Part model, mm, in its own coordinate system. Round coordinates to 2 decimals unless told otherwise and drop trailing zeros. Write each loop counter-clockwise with the first axis right and the second up, starting at its lowest first coordinate (ties: lowest second). Pieces come first, ordered by that corner, then holes. Notation, with made-up numbers: (-20, -16.5) -> (21, -16.5) arc R34 cw to (21, 15.5) -> close; hole circle Ø10 at (39, 57.5). An arc over 180 degrees is marked (long way). Return JSON: item names as keys, results as strings. Group by question number.
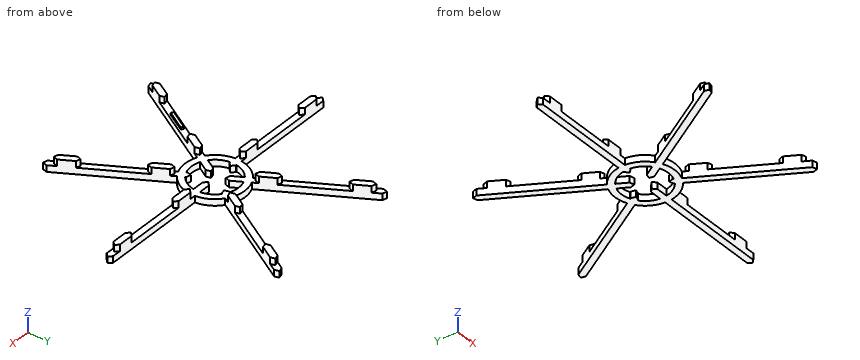
```python
from build123d import *

# Parameters (mm, degrees)
F1_DEPTH = 3
F4_DEPTH = 3
F5_COUNT = 3
F5_ANGLE = 240
F7_DEPTH = 1
F8_R     = 14
F8_R_2   = 11
F9_DEPTH = 3


# Not quite as in the source:
# - a feature names something its author has since deleted; it is built from what else it names


with BuildPart() as f1:
    # F0 (on Top) → F1 (new body)
    with BuildSketch(Plane.XY):
        Polygon((-2, -3.4641016151), (-4.0490381057, -4.0131397208), (-32.5490381057, -53.3765877365), (-32, -55.4256258422), (-29.9509618943, -54.8765877365), (-1.4509618943, -5.5131397208), align=None)
    extrude(amount=F1_DEPTH)

    # F3 (on face) → F4, piece 2 (join)
    with BuildSketch(Plane.XY.offset(3)):
        Polygon((-27.0490381057, -43.8503082949), (-30.5490381057, -49.9124861214), (-30, -51.9615242271), (-27.9509618943, -51.4124861214), (-24.4509618943, -45.3503082949), (-25, -43.3012701892), align=None)
        Polygon((-9.5490381057, -13.5394191624), (-13.0490381057, -19.6015969889), (-12.5, -21.6506350946), (-10.4509618943, -21.1015969889), (-6.9509618943, -15.0394191624), (-7.5, -12.9903810568), align=None)
    extrude(amount=F4_DEPTH)


with BuildPart() as f1b:
    # F0 (on Top) → F1, piece 2 (new body)
    with BuildSketch(Plane.XY):
        Polygon((-10.5, 1.5), (-62.5, 1.5), (-64, 0), (-62.5, -1.5), (-10.5, -1.5), (-9, 0), align=None)
    extrude(amount=F1_DEPTH)

    # F3 (on face) → F4 (join)
    with BuildSketch(Plane.XY.offset(3)):
        Polygon((-51.5, 1.5), (-58.5, 1.5), (-60, 0), (-58.5, -1.5), (-51.5, -1.5), (-50, 0), align=None)
        Polygon((-16.5, 1.5), (-23.5, 1.5), (-25, 0), (-23.5, -1.5), (-16.5, -1.5), (-15, 0), align=None)
    extrude(amount=F4_DEPTH)


with BuildPart() as f5_1:
    # F5: instance of F1
    add(f1.part.rotate(Axis((0, 0, 0.1916177571), (0, 0, -1)), 1 * F5_ANGLE / (F5_COUNT - 1)))


with BuildPart() as f5_2:
    # F5: instance of F1
    add(f1.part.rotate(Axis((0, 0, 0.1916177571), (0, 0, -1)), 2 * F5_ANGLE / (F5_COUNT - 1)))


with BuildPart() as f5_3:
    # F5: instance of F1b
    add(f1b.part.rotate(Axis((0, 0, 0.1916177571), (0, 0, -1)), 1 * F5_ANGLE / (F5_COUNT - 1)))


with BuildPart() as f5_4:
    # F5: instance of F1b
    add(f1b.part.rotate(Axis((0, 0, 0.1916177571), (0, 0, -1)), 2 * F5_ANGLE / (F5_COUNT - 1)))


with BuildPart() as f1_1:
    add(f1.part)

    # F6 (on face) → F7 (join)
    with BuildSketch(Plane.XY.offset(3)):
        Polygon((-15.7303847577, -28.445825623), (-16.7696152423, -27.845825623), (-21.7696152423, -36.5060796608), (-20.7303847577, -37.1060796608), align=None)
    extrude(amount=F7_DEPTH)

    add(f1b.part)  # F9 merges F1b

    add(f5_1.part)  # F9 merges F5_1

    add(f5_2.part)  # F9 merges F5_2

    add(f5_3.part)  # F9 merges F5_3

    add(f5_4.part)  # F9 merges F5_4
    # F8 (on Top) → F9 (join)
    with BuildSketch(Plane.XY):
        Circle(F8_R)
        Circle(F8_R_2, mode=Mode.SUBTRACT)
    extrude(amount=F9_DEPTH)


solid = f1_1.part
```
Item 1: Cut at B-B (y = -41). Write the cut outline in (x, z).
Item 2: Flat gauge pins, fed straight in: P1, Ø8.5, axis at x = 20, y = -37.5, coming from the +Z side; P2, Ø3, axis at x = 39, z = 4, coming from the -Y side; P3, Ø2.5, axis at x = 9, z = 2, coming from the +Y side. Where does each tip first touch, or does it go through?
Item 3: Wall check: L1, parallel to Y at x = 31, z = 2.1; L2, parallel to Y at x = 58, z = 4.55; L3, parallel to Y at x = -0.5, z = 0.55. Give the ranges that are in metal, low to high.
Item 4: Cut at A-A (x = 1). Write the cut outline in (y, z), then the cut area to 3 significant figures.
Checks:
{
 "1": {"outline": "(-25.4, 0) -> (-21.94, 0) -> (-21.94, 3) -> (-25.4, 3) -> close; (21.94, 0) -> (25.4, 0) -> (25.4, 3) -> (21.94, 3) -> close"},
 "2": {"P1": "stops at z = 3", "P2": "stops at y = -1.5", "P3": "stops at y = 20.75"},
 "3": {"L1": "y = -55.16 to -50.69, -1.5 to 1.5, 50.69 to 55.16", "L2": "y = -1.5 to 1.5", "L3": "y = -13.99 to -10.99, 10.99 to 13.99"},
 "4": {"outline": "(-13.96, 0) -> (-10.95, 0) -> (-10.95, 3) -> (-13.96, 3) -> close; (10.95, 0) -> (13.96, 0) -> (13.96, 3) -> (10.95, 3) -> close", "area": "18.1 mm2"}
}
